```python
from build123d import *

# Parameters (mm, degrees)
SKETCH1_W               = 60
SKETCH1_H               = 40
BOSS_EXTRUDE1_DEPTH     = 20
CUT_EXTRUDE1_DEPTH      = 30
SKETCH3_W               = 60
SKETCH3_H               = 15
BOSS_EXTRUDE2_DEPTH     = 40
SKETCH4_R               = 2.1
CUT_EXTRUDE2_DEPTH      = 20
FILLET1_R               = 2
FILLET2_R               = 2
ESQUISSE1_W             = 40
ESQUISSE1_H             = 30
ENL_V_MAT_EXTRU_1_DEPTH = 16.5
CONG_1_R                = 1


with BuildPart() as part:
    # Sketch1 → Boss-Extrude1 (new body)
    with BuildSketch(Plane.XY):
        with Locations((5, -2.5)):
            Rectangle(SKETCH1_W, SKETCH1_H)
    extrude(amount=BOSS_EXTRUDE1_DEPTH)

    # Sketch2 → Cut-Extrude1 (cut)
    with BuildSketch(Plane.XY.offset(20)):
        with BuildLine():
            ThreePointArc((-7.574074074, -7.413518208), (5, -16), (17.574074074, -7.413518208))
            ThreePointArc((17.574074074, -7.413518208), (23.5, -2.5), (17.574074074, 2.413518208))
            ThreePointArc((17.574074074, 2.413518208), (5, 11), (-7.574074074, 2.413518208))
            ThreePointArc((-7.574074074, 2.413518208), (-13.5, -2.5), (-7.574074074, -7.413518208))
        make_face()
    extrude(amount=-CUT_EXTRUDE1_DEPTH, mode=Mode.SUBTRACT)

    # Sketch3 → Boss-Extrude2 (add)
    with BuildSketch(Plane(origin=(0, 0, 0), x_dir=(-1, 0, 0), z_dir=(0, 0, -1))):
        with Locations((-5, -30)):
            Rectangle(SKETCH3_W, SKETCH3_H)
    extrude(amount=-BOSS_EXTRUDE2_DEPTH)

    # Sketch4 → Cut-Extrude2 (cut)
    with BuildSketch(Plane(origin=(0, -22.5, 0), x_dir=(1, 0, 0), z_dir=(0, 1, 0))):
        with Locations(Location((-18, -35, 0), (0, 0, 180))):
            Circle(SKETCH4_R)
        with Locations(Location((-18, -25, 0), (0, 0, 180))):
            Circle(SKETCH4_R)
        with Locations(Location((28, -35, 0), (0, 0, 180))):
            Circle(SKETCH4_R)
        with Locations(Location((28, -25, 0), (0, 0, 180))):
            Circle(SKETCH4_R)
    extrude(amount=-CUT_EXTRUDE2_DEPTH, mode=Mode.SUBTRACT)

    # Fillet1
    fillet1_edges = [part.edges().sort_by_distance(p)[0] for p in [
        (5, -22.5, 20),
    ]]
    fillet(fillet1_edges, radius=FILLET1_R)

    # Fillet2
    fillet2_edges = [part.edges().sort_by_distance(p)[0] for p in [
        (35, -30, 40),
        (-25, -30, 40),
        (5, -37.5, 0),
        (-25, 17.5, 10),
        (35, 17.5, 10),
    ]]
    fillet(fillet2_edges, radius=FILLET2_R)

    # Esquisse1 → Enlèv. mat.-Extru.1 (cut)
    with BuildSketch(Plane.XY.offset(20)):
        with Locations((5, -2.5)):
            Rectangle(ESQUISSE1_W, ESQUISSE1_H)
    extrude(amount=-ENL_V_MAT_EXTRU_1_DEPTH, mode=Mode.SUBTRACT)

    # Congé1
    cong_1_edges = [part.edges().sort_by_distance(p)[0] for p in [
        (-15, -2.5, 20),
        (5, -17.5, 20),
        (25, -2.5, 20),
        (5, 12.5, 20),
        (-15, -2.5, 3.5),
        (-15, -17.5, 11.75),
        (5, 12.5, 3.5),
        (-15, 12.5, 11.75),
        (25, -2.5, 3.5),
        (25, 12.5, 11.75),
        (5, -17.5, 3.5),
        (25, -17.5, 11.75),
        (35, -2.5, 20),
        (35, -21.914213562, 20.585786438),
        (-25, -21.914213562, 20.585786438),
        (-25, -22.5, 30),
        (-25, -2.5, 20),
        (35, -22.5, 30),
        (5, -22.5, 40),
        (-24.414213562, -22.5, 39.414213562),
        (34.414213562, -22.5, 39.414213562),
        (5, 17.5, 20),
        (34.414213562, 16.914213562, 20),
        (-24.414213562, 16.914213562, 20),
    ]]
    fillet(cong_1_edges, radius=CONG_1_R)


solid = part.part
```
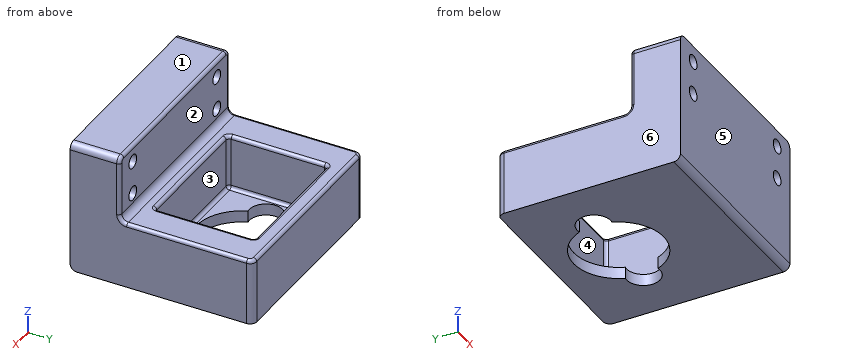
Work out the finished part from the listing and answer in its coordinate system (mm). Face numbers are marked on the shaded views. A direction names the side the tool comes from. Give positions to 0.01 mm unless a question says otherwise; leave off trailing zeros. Write each loop counter-clockwise with the first axis right and the second up, starting at its lowest first coordinate (ties: lowest second). Pieces come first, ordered by that corner, then holes. Notation, with made-up numbers: (17.5, 3) -> (50.5, 3) arc R33 cw to (50.5, 32) -> close; hole circle Ø11 at (85.25, 7.25). An arc over 180 degrees is marked (long way). Write each question's results on one line, items separated by ' | '.
1. Determine the mould class of the marked faces 4, 5 and 6 for opening direction Y: +Y half, -Y half, draft (parallel to the pull), parting line (faces both ways), or undercut.
Data:
face 4: undercut | face 5: -Y half | face 6: draft
2. Find section C-C on z = 14.5. Determine the outline of the cut face in (x, y).
Data:
outline: (-25, -37.5) -> (35, -37.5) -> (35, 15.5) arc R2 ccw to (33, 17.5) -> (-23, 17.5) arc R2 ccw to (-25, 15.5) -> close; hole (-15, -16.5) arc R1 ccw to (-14, -17.5) -> (24, -17.5) arc R1 ccw to (25, -16.5) -> (25, 11.5) arc R1 ccw to (24, 12.5) -> (-14, 12.5) arc R1 ccw to (-15, 11.5) -> close
3. Each of these flat-tipped pins is pushed along its axis until it touches: pin 1 Ø16 at (x, y) = (-8.5, -2.5) entering from +Z; pin 2 Ø6.5 at (x, z) = (-18, 25) entering from +Y; pin 3 Ø3.5 at (x, z) = (28, 25) entering from -Y; pin 4 Ø6 at (x, y) = (-2.5, 8.5) entering from +Z. Where does it stop, or does it pass through?
Data:
pin 1: z = 20 | pin 2: y = -22.48 | pin 3: through | pin 4: z = 3.5
4. Straight lines are drawn through the part: L1, parallel to Z at x = 28, y = -28; L2, parallel to Y at x = 2, z = 9; L3, parallel to X at y = -11.5, z = 16. For each, find the intervals that lie inside material, in ascending order.
Data:
L1: 0 to 22.9, 27.1 to 32.9, 37.1 to 40 | L2: -37.5 to -17.5, 12.5 to 17.5 | L3: -25 to -15, 25 to 35
5. Find section A-A on x = -18. Determine the outline of the cut face in (y, z).
Data:
outline: (-37.5, 2) arc R2 ccw to (-35.5, 0) -> (17.5, 0) -> (17.5, 19) arc R1 ccw to (16.5, 20) -> (-20.5, 20) arc R2 cw to (-22.5, 22) -> (-22.5, 22.9) -> (-37.5, 22.9) -> close; (-37.5, 27.1) -> (-22.5, 27.1) -> (-22.5, 32.9) -> (-37.5, 32.9) -> close; (-37.5, 37.1) -> (-22.5, 37.1) -> (-22.5, 39) arc R1 ccw to (-23.5, 40) -> (-37.5, 40) -> close
6. Find section D-D on y = -26.5. Determine the outline of the cut face in (x, z), and give its area (3 significant figures).
Data:
outline: (-25, 0) -> (35, 0) -> (35, 38) arc R2 ccw to (33, 40) -> (-23, 40) arc R2 ccw to (-25, 38) -> close; hole circle Ø4.2 at (-18, 25); hole circle Ø4.2 at (-18, 35); hole circle Ø4.2 at (28, 25); hole circle Ø4.2 at (28, 35) | area: 2,340 mm^2
7. Find section B-B on y = 1.5. Determine the outline of the cut face in (x, z), and give its area (3 significant figures).
Data:
outline: (-25, 0) -> (-11.5, 0) -> (-11.5, 3.5) -> (-14, 3.5) arc R1 cw to (-15, 4.5) -> (-15, 19) arc R1 ccw to (-16, 20) -> (-24, 20) arc R1 ccw to (-25, 19) -> close; (21.5, 0) -> (35, 0) -> (35, 19) arc R1 ccw to (34, 20) -> (26, 20) arc R1 ccw to (25, 19) -> (25, 4.5) arc R1 cw to (24, 3.5) -> (21.5, 3.5) -> close | area: 424 mm^2
8. A tool of negligible diameter and unlimited length cuts with its end or side. For the marked faces 1, 2 and 3, from which of +Z, -Z, +X, -X, +Y, -Y can it reach the whole face along a straight path? Write none if from no direction.
Data:
face 1: +Z, +X, -X, +Y, -Y | face 2: +Z, +X, -X, +Y | face 3: +Z
